Build history of the part. All positions in model axes, mm. A direction names the side the tool comes from. Round coordinates to 2 decimals unless told otherwise and drop trailing zeros. Order: outer loops, then holes, each group sorted by start corner. A loop starts at its lowest first (then second) coordinate and runs counter-clockwise, first axis right, second up. Notation, with made-up numbers: M 84.25,62 L 91.25,62 A16 ccw 91.25,77 Z; hole C 76.25,6.25 d9. An arc over 180 degrees is marked long. One line per item, written item: value. Start each with the question number.
Item 1: Band-saw the part on B-B, the plane x = 0. Give the number of separate pieces and of enclosed holes in the cut face, then the cut area to 3 significant figures.
Item 2: Tool access for faces 4 (the cylindrical face through (-1.08, 40.38, 4.93)), 5 (the flat face through (9, 9, 10)): list every direction of +Z, -Z, +X, -X, +Y, -Y with a clear straight run to the whole face (end or side of a thin tool).
Item 3: Pin check, flat tips, straight feed: pin 1 (1 mm diameter, centred on y = -15, z = 6, fed in from -X); pin 2 (2 mm diameter, centred on x = -14.5, y = -13, fed in from +Z); pin 3 (8 mm diameter, centred on x = 15, z = 6.5, fed in from -Y). Stop position of each tip, or through.
Item 4: Two-plate mould, pull along X, no slides. Class faces 1 (the flat face through (7, 19, 4)), 2 (the flat face through (0, 11, 0)), 3 (the cylindrical face through (0, -45, 5)): +X half, -X half, draft (parallel to the pull), parting line (faces both ways), or undercut.
Item 5: Band-saw the part on C-C, the plane y = -35.5. Write the cut outline in (x, z), then the cut area to 3 significant figures.
Item 6: Band-saw the part on D-D, the plane y = 28. Write the cut outline in (x, z).
Item 7: Band-saw the part on A-A, the plane y = 0. Write the cut outline in (x, z).
Item 8: Probe L1, parallel to Y at x = 3, z = 9.5; L2, parallel to X at y = 12, z = 8; L3, parallel to Y at x = -12, z = 7. List the from-to ranges inside material, lowest first.
Autodesk Inventor part; units mm, degrees
ref_plane "YZ Plane" through (0, 0, 0) normal (1, 0, 0) x (0, 1, 0)
ref_plane "XZ Plane" through (0, 0, 0) normal (0, 1, 0) x (-1, 0, 0)
ref_plane "XY Plane" through (0, 0, 0) normal (0, 0, 1) x (1, 0, 0)
sketch "Sketch1" plane through (0, 0, 0) normal (0, 0, 1) x (1, 0, 0)
  circle A0 centre (0, 0) radius 10
  circle A1 centre (0, 35.5) radius 5
  circle A2 centre (0, -35.5) radius 5
  circle A3 centre (0, -35.5) radius 9.5
  circle A4 centre (0, 35.5) radius 9.5
  circle A5 centre (0, 0) radius 25
  circle A6 centre (0, 0) radius 20
  line L0 (-23.7028, 13.9437) -> (-8.1883, 40.3169)
  line L1 (8.1883, 40.3169) -> (23.7028, 13.9437)
  line L2 (8.1883, -40.3169) -> (23.7028, -13.9437)
  line L3 (-8.1883, -40.3169) -> (-23.7028, -13.9437)
  arc A7 (-4.4942, 27.1303) -> (-4.4942, -27.1303) centre (0, 0) ccw
  arc A8 (4.4942, -27.1303) -> (4.4942, 27.1303) centre (0, 0) ccw
  dimension "d0" = 20
  dimension "d4" = 10
  dimension "d5" = 10
  dimension "d7" = 19
  dimension "d8" = 50
  dimension "d9" = 40
extrude "Extrusion1" add sketch "Sketch1" along normal blind 10
sketch "Sketch2" plane through (0, 0, 10) normal (0, 0, 1) x (1, 0, 0)
  circle A0 centre (0, 0) radius 10
  circle A1 centre (0, 0) radius 12.5
  dimension "d14" = 25
extrude "Extrusion2" add sketch "Sketch2" along normal blind 4
sketch "Sketch3" plane through (0, 0, 0) normal (0, 0, -1) x (-1, 0, 0)
  circle A0 centre (0, 0) radius 20
  circle A1 centre (0, 0) radius 25
extrude "Extrusion3" add sketch "Sketch3" against normal blind 4
fillet "Fillet1" radius 2 1 edges at (-25, 0, 4)
properties part number "bearing"
Output:
1. separate pieces: 4
1. enclosed holes: 0
1. area: 462 mm²
2. face 4: +Z, -Z
2. face 5: +Z
3. pin 1: stops at x = -23.38
3. pin 2: stops at z = 10
3. pin 3: stops at y = -35.54
4. face 1: undercut
4. face 2: draft
4. face 3: parting line
5. outline: M -11.02,0 L -5,0 L -5,10 L -11.02,10 Z; M 5,0 L 11.02,0 L 11.02,10 L 5,10 Z
5. area: 120 mm²
6. outline: M -15.43,0 L 15.43,0 L 15.43,10 L -15.43,10 Z
7. outline: M -27.5,0 L -10,0 L -10,14 L -12.5,14 L -12.5,10 L -20,10 L -20,4 L -23,4 A2 cw -25,6 L -25,10 L -27.5,10 Z; M 10,0 L 27.5,0 L 27.5,10 L 25,10 L 25,6 A2 cw 23,4 L 20,4 L 20,10 L 12.5,10 L 12.5,14 L 10,14 Z
8. L1: y = -44.51 to -39.5, -31.5 to -24.82, -19.77 to -9.54, 9.54 to 19.77, 24.82 to 31.5, 39.5 to 44.51
8. L2: x = -24.74 to -21.93, -16 to 16, 21.93 to 24.74
8. L3: y = -33.84 to -21.93, -16 to 16, 21.93 to 33.84
